Geometry: final body of the model. Coordinates: model frame, mm. A direction names the side the tool comes from. Give positions to 0.01 mm unless a question says otherwise; leave off trailing zeros. Write each loop counter-clockwise with the first axis right and the second up, starting at its lowest first coordinate (ties: lowest second). Pieces come first, ordered by that corner, then holes.
from build123d import *

# Parameters (mm, degrees)
BOSS_EXTRUDE1_DEPTH = 149


with BuildPart() as part:
    # Sketch1 → Boss-Extrude1 (new body)
    with BuildSketch(Plane.XY):
        with BuildLine():
            Line((-11.199951579, -12.7), (-4.222256762, -12.7))
            ThreePointArc((-4.222256762, -12.7), (-3.503836272, -12.40242049), (-3.206256762, -11.684))
            Line((-3.206256762, -11.684), (-3.206256762, -11.440665395))
            ThreePointArc((-3.206256762, -11.440665395), (-3.503836272, -10.722244905), (-4.222256762, -10.424665395))
            Line((-4.222256762, -10.424665395), (-6.40926672, -10.424665395))
            ThreePointArc((-6.40926672, -10.424665395), (-7.347928334, -9.797471742), (-7.127687178, -8.690244874))
            Line((-7.127687178, -8.690244874), (-3.593166694, -5.155724698))
            ThreePointArc((-3.593166694, -5.155724698), (-2.876257435, -4.67670128), (-2.030605322, -4.508490626))
            Line((-2.030605322, -4.508490626), (2.030598864, -4.508490626))
            ThreePointArc((2.030598864, -4.508490626), (2.876251031, -4.676701303), (3.593160319, -5.155724782))
            Line((3.593160319, -5.155724782), (7.127680379, -8.690244912))
            ThreePointArc((7.127680379, -8.690244912), (7.347921489, -9.019859032), (7.425259882, -9.408665395))
            ThreePointArc((7.425259882, -9.408665395), (7.127680372, -10.127085884), (6.409259882, -10.424665395))
            Line((6.409259882, -10.424665395), (4.22225065, -10.424665395))
            ThreePointArc((4.22225065, -10.424665395), (3.50383016, -10.722244905), (3.20625065, -11.440665395))
            Line((3.20625065, -11.440665395), (3.20625065, -11.684))
            ThreePointArc((3.20625065, -11.684), (3.50383016, -12.40242049), (4.22225065, -12.7))
            Line((4.22225065, -12.7), (11.199952422, -12.7))
            Line((11.199952422, -12.7), (12.7, -11.199951732))
            Line((12.7, -11.199951732), (12.7, -4.222256762))
            ThreePointArc((12.7, -4.222256762), (12.40242049, -3.503836272), (11.684, -3.206256762))
            Line((11.684, -3.206256762), (11.440665395, -3.206256762))
            ThreePointArc((11.440665395, -3.206256762), (10.722244905, -3.503836272), (10.424665395, -4.222256762))
            Line((10.424665395, -4.222256762), (10.424665395, -6.40926672))
            ThreePointArc((10.424665395, -6.40926672), (9.797471742, -7.347928334), (8.690244874, -7.127687178))
            Line((8.690244874, -7.127687178), (5.155724698, -3.593166694))
            ThreePointArc((5.155724698, -3.593166694), (4.67670128, -2.876257435), (4.508490626, -2.030605322))
            Line((4.508490626, -2.030605322), (4.508490626, 2.030598864))
            ThreePointArc((4.508490626, 2.030598864), (4.676701303, 2.876251031), (5.155724782, 3.593160319))
            Line((5.155724782, 3.593160319), (8.690244912, 7.127680379))
            ThreePointArc((8.690244912, 7.127680379), (9.019859032, 7.347921489), (9.408665395, 7.425259882))
            ThreePointArc((9.408665395, 7.425259882), (10.127085884, 7.127680372), (10.424665395, 6.409259882))
            Line((10.424665395, 6.409259882), (10.424665395, 4.22225065))
            ThreePointArc((10.424665395, 4.22225065), (10.722244905, 3.50383016), (11.440665395, 3.20625065))
            Line((11.440665395, 3.20625065), (11.684, 3.20625065))
            ThreePointArc((11.684, 3.20625065), (12.40242049, 3.50383016), (12.7, 4.22225065))
            Line((12.7, 4.22225065), (12.7, 11.199954756))
            Line((12.7, 11.199954756), (11.199954423, 12.7))
            Line((11.199954423, 12.7), (4.222256762, 12.7))
            ThreePointArc((4.222256762, 12.7), (3.503836272, 12.40242049), (3.206256762, 11.684))
            Line((3.206256762, 11.684), (3.206256762, 11.440665395))
            ThreePointArc((3.206256762, 11.440665395), (3.503836272, 10.722244905), (4.222256762, 10.424665395))
            Line((4.222256762, 10.424665395), (6.40926672, 10.424665395))
            ThreePointArc((6.40926672, 10.424665395), (7.347928334, 9.797471742), (7.127687178, 8.690244874))
            Line((7.127687178, 8.690244874), (3.593166694, 5.155724698))
            ThreePointArc((3.593166694, 5.155724698), (2.876257435, 4.67670128), (2.030605322, 4.508490626))
            Line((2.030605322, 4.508490626), (-2.030598864, 4.508490626))
            ThreePointArc((-2.030598864, 4.508490626), (-2.876251031, 4.676701303), (-3.593160319, 5.155724782))
            Line((-3.593160319, 5.155724782), (-7.127680379, 8.690244912))
            ThreePointArc((-7.127680379, 8.690244912), (-7.347921489, 9.019859032), (-7.425259882, 9.408665395))
            ThreePointArc((-7.425259882, 9.408665395), (-7.127680372, 10.127085884), (-6.409259882, 10.424665395))
            Line((-6.409259882, 10.424665395), (-4.22225065, 10.424665395))
            ThreePointArc((-4.22225065, 10.424665395), (-3.50383016, 10.722244905), (-3.20625065, 11.440665395))
            Line((-3.20625065, 11.440665395), (-3.20625065, 11.684))
            ThreePointArc((-3.20625065, 11.684), (-3.50383016, 12.40242049), (-4.22225065, 12.7))
            Line((-4.22225065, 12.7), (-11.199951733, 12.7))
            Line((-11.199951733, 12.7), (-12.7, 11.1999514))
            Line((-12.7, 11.1999514), (-12.7, 4.222256762))
            ThreePointArc((-12.7, 4.222256762), (-12.40242049, 3.503836272), (-11.684, 3.206256762))
            Line((-11.684, 3.206256762), (-11.440665395, 3.206256762))
            ThreePointArc((-11.440665395, 3.206256762), (-10.722244905, 3.503836272), (-10.424665395, 4.222256762))
            Line((-10.424665395, 4.222256762), (-10.424665395, 6.40926672))
            ThreePointArc((-10.424665395, 6.40926672), (-9.797471742, 7.347928334), (-8.690244874, 7.127687178))
            Line((-8.690244874, 7.127687178), (-5.155724698, 3.593166694))
            ThreePointArc((-5.155724698, 3.593166694), (-4.67670128, 2.876257435), (-4.508490626, 2.030605322))
            Line((-4.508490626, 2.030605322), (-4.508490626, -2.030598864))
            ThreePointArc((-4.508490626, -2.030598864), (-4.676701303, -2.876251031), (-5.155724782, -3.593160319))
            Line((-5.155724782, -3.593160319), (-8.690244912, -7.127680379))
            ThreePointArc((-8.690244912, -7.127680379), (-9.019859032, -7.347921489), (-9.408665395, -7.425259882))
            ThreePointArc((-9.408665395, -7.425259882), (-10.127085884, -7.127680372), (-10.424665395, -6.409259882))
            Line((-10.424665395, -6.409259882), (-10.424665395, -4.22225065))
            ThreePointArc((-10.424665395, -4.22225065), (-10.722244905, -3.50383016), (-11.440665395, -3.20625065))
            Line((-11.440665395, -3.20625065), (-11.684, -3.20625065))
            ThreePointArc((-11.684, -3.20625065), (-12.40242049, -3.50383016), (-12.7, -4.22225065))
            Line((-12.7, -4.22225065), (-12.7, -11.199952268))
            Line((-12.7, -11.199952268), (-11.199951579, -12.7))
        make_face()
        with BuildLine():
            ThreePointArc((-2.55499489, 0), (0, -2.55499489), (2.55499489, 0))
            ThreePointArc((2.55499489, 0), (0, 2.55499489), (-2.55499489, 0))
        make_face(mode=Mode.SUBTRACT)
    extrude(amount=BOSS_EXTRUDE1_DEPTH)


solid = part.part
Q1. Access query for faces 4 (the flat face through (-5.34, 6.9, 73.46)), 5 (the flat face through (0, 4.508, 73)), 6 (the flat face through (0, -4.508, 73)), 7 (the flat face through (4.508, 0, 73)). Directions: +Z, -Z, +X, -X, +Y, -Y. A direction counts if a zero-diameter tool reaches every point of the face in a straight line with its end or side. Return the directions, or none.
Filled sheet:
face 4: +Z, -Z
face 5: +Z, -Z, +Y
face 6: +Z, -Z, -Y
face 7: +Z, -Z, +X
Q2. Ray query, line 1 along Y through (x, z) = (-5.5, 132); line 2 along Y through (x, z) = (0, 104.5) (1 decimal); line 3 along X through (y, z) = (-5, 21.5). Return the intervals inside material, ascending.
Filled sheet:
line 1: y = -12.7 to -10.42, -7.06 to -3.94, 3.94 to 7.06, 10.42 to 12.7
line 2: y = -4.5 to -2.6, 2.6 to 4.5
line 3: x = -12.7 to -10.42, -6.56 to -3.42, 3.42 to 6.56, 10.42 to 12.7
Q3. Section A-A on y = 0. Output: boundary loops of the cut face in (x, z) (1 decimal).
Filled sheet:
outline: (-4.5, 0) - (-2.6, 0) - (-2.6, 149) - (-4.5, 149) - close; (2.6, 0) - (4.5, 0) - (4.5, 149) - (2.6, 149) - close
Q4. Pin query (flat end, axial travel): P1, Ø4.5, axis at x = 0, z = 78, coming from the +Y side; P2, Ø3, axis at y = 0.5, z = 52.5, coming from the -X side; P3, Ø4, axis at y = 1.5, z = 97.5, coming from the -X side. Return the tip coordinate at first contact, or that it passes through.
Filled sheet:
P1: stops at y = 4.52
P2: stops at x = -4.51
P3: stops at x = -12.4
Q5. Pull-direction query (Y, two-part tool) for faces 1 (the flat face through (12.7, -8, 73)), 2 (the flat face through (6.95, -5.39, 73.46)), 3 (the flat face through (8, 12.7, 73)); classes: released by +Y, released by -Y, zero draft, split by the parting line, or undercut.
Filled sheet:
face 1: zero draft
face 2: undercut
face 3: released by +Y
